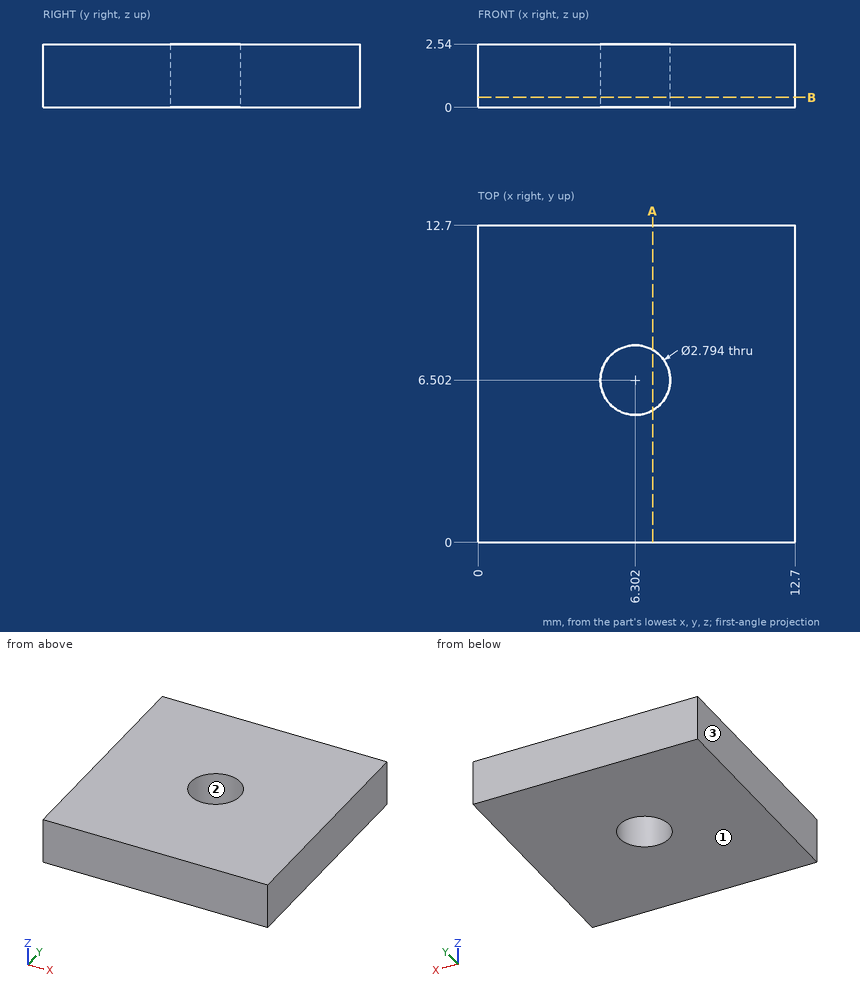
Geometry check sheet. Reference: drawing and pictorial views, mm from the part's lowest x, y, z. Give positions to 0.01 mm unless a question says otherwise; leave off trailing zeros. Order: outer loops, then holes, each group sorted by start corner. A loop starts at its lowest first (then second) coordinate and runs counter-clockwise, first axis right, second up. Notation, with made-up numbers: M 19,0.25 L 30,0.25 A32 cw 30,28.25 Z; hole C 29,61.25 d6. An arc over 180 degrees is marked long. Answer in a Markdown table with one row per item. Add a question column.
Q1. Sectioned sample at B-B, the plane z = 0.4. Record the boundary of the cut face in (x, y).
Q2. Gauge pin test, flat end, axial feed: pin 1 Ø2 at (x, y) = (6.3, 6.5) entering from -Z. Record the tip position at first contact, or that the pin passes through.
Q3. Release check for a two-part mould opening along X. For the marked faces 1, 2 and 3 record: released by +X, released by -X, zero draft, split by the parting line, or undercut.
Q4. Thickness scan on L1, parallel to Y at x = 7, z = 1.8; L2, parallel to X at y = 5.5, z = 2.1 (1 decimal); L3, parallel to Y at x = 5.25, z = 1.85. Record the ranges inside material, lowest first.
Q5. Sectioned sample at A-A, the plane x = 7. Record the boundary of the cut face in (y, z).
Verdict:
| question | item | result |
|---|---|---|
| 1 | outline | M 0,0 L 12.7,0 L 12.7,12.7 L 0,12.7 Z; hole C 6.3,6.5 d2.79 |
| 2 | pin 1 | through |
| 3 | face 1 | zero draft |
| 3 | face 2 | undercut |
| 3 | face 3 | released by -X |
| 4 | L1 | 0 to 5.29, 7.71 to 12.7 |
| 4 | L2 | 0 to 5.3, 7.3 to 12.7 |
| 4 | L3 | 0 to 5.58, 7.42 to 12.7 |
| 5 | outline | M 0,0 L 5.29,0 L 5.29,2.54 L 0,2.54 Z; M 7.71,0 L 12.7,0 L 12.7,2.54 L 7.71,2.54 Z |
